Source: CAD feature listing. Evaluate the final solid. Frame: model axes, mm. A direction names the side the tool comes from. Give positions to 0.01 mm unless a question says otherwise; leave off trailing zeros. Write item = value, one per line.
from build123d import *

# Parameters (mm, degrees)
BOSS_EXTRUDE1_DEPTH = 63
CUT_EXTRUDE4_DEPTH  = 60
BOSS_EXTRUDE5_DEPTH = 5
FILLET3_R           = 5
BOSS_EXTRUDE6_DEPTH = 5
BOSS_EXTRUDE7_DEPTH = 63
FILLET4_R           = 5
SKETCH14_R          = 1.9999999999999996
SKETCH14_R_2        = 2
CUT_EXTRUDE5_DEPTH  = 10
SKETCH15_R          = 4.000000000000002
SKETCH15_R_2        = 2
SKETCH15_R_3        = 4.000000000000001
SKETCH15_R_4        = 1.9999999999999996
BOSS_EXTRUDE8_DEPTH = 5
CUT_EXTRUDE6_START  = -5
SKETCH16_R          = 2
SKETCH16_R_2        = 1.9999999999999996
CUT_EXTRUDE6_DEPTH  = 5


# Read off the part's stored shape, not the designer's step: Boss-Extrude1
with BuildPart() as part:
    # Boss-Extrude1 outline → Boss-Extrude1 (new body)
    with BuildSketch(Plane.XY):
        with BuildLine():
            Line((4.954113003, -60.810475982), (9.954113003, -60.810475982))
            add(Edge.make_bspline(
                [(9.954113003, -60.810475982), (1.78782004145555, -34.5665002552168), (-27.9913048539535, -7.28206006884536), (-18.045886997, 21.189524018)],
                knots=[0, 0, 0, 0, 1, 1, 1, 1], degree=3))
            Line((-18.045886997, 21.189524018), (-23.045886997, 21.189524018))
            add(Edge.make_bspline(
                [(-23.045886997, 21.189524018), (-23.192896954450642, 20.707388183877445), (-23.619107908159766, 19.212032019757164), (-24.3984566732412, 15.7227335791878), (-24.9259424602794, 10.7154717202631), (-24.7059244457818, 4.80639957244901), (-23.4437954980132, -2.90791828688786), (-20.3649701079, -12.2138739410152), (-15.1627192062184, -22.9267758821705), (-9.22446854976525, -33.2839412268649), (-4.2731817504284, -41.6523064711653), (-0.670405229165687, -48.1782991582584), (1.76514247549924, -52.980809675903), (3.49961876568494, -56.8892897902748), (4.492016037450547, -59.4867262662843), (4.856824135774904, -60.5259563871115), (4.954113003, -60.810475982)],
                knots=[0.01630237867055594, 0.01630237867055594, 0.01630237867055594, 0.01630237867055594, 0.03125, 0.0625, 0.125, 0.1875, 0.25, 0.375, 0.5, 0.625, 0.75, 0.8125, 0.875, 0.9375, 0.96875, 0.9805431413660037, 0.9805431413660037, 0.9805431413660037, 0.9805431413660037], degree=3))
        make_face()
    extrude(amount=BOSS_EXTRUDE1_DEPTH)

    # Sketch10 → Cut-Extrude4 (cut)
    with BuildSketch(Plane.XZ.offset(60.81047598214444)):
        with BuildLine():
            Line((9.954113003304059, 63), (9.954113003304059, 44.66190378968828))
            ThreePointArc((9.954113003304059, 44.66190378968828), (4.065539070195477, 55.13527900478137), (-5.018130619372688, 63))
            Line((-5.018130619372688, 63), (4.954113003304057, 63))
            Line((4.954113003304057, 63), (9.954113003304059, 63))
        make_face()
    extrude(amount=-CUT_EXTRUDE4_DEPTH, mode=Mode.SUBTRACT)

    # Sketch11 → Boss-Extrude5 (add)
    with BuildSketch(Plane.XZ.offset(60.81047598214444)):
        with BuildLine():
            Line((-15.045886996695936, 6e-16), (4.954113003304057, 0))
            Line((4.954113003304057, 0), (4.954113003304058, 54.00000000000057))
            ThreePointArc((4.954113003304058, 54.00000000000057), (0.4038163976446967, 58.98290612532635), (-5.018130619372695, 63))
            Line((-5.018130619372695, 63), (-15.045886996695936, 63))
            Line((-15.045886996695936, 63), (-15.045886996695936, 6e-16))
        make_face()
    extrude(amount=-BOSS_EXTRUDE5_DEPTH)

    # Fillet3
    fillet3_edges = [part.edges().sort_by_distance(p)[0] for p in [
        (3.003762593217399, -55.81047598214444, 28.187768789799662),
    ]]
    fillet(fillet3_edges, radius=FILLET3_R)



with BuildPart() as body_2:
    # Sketch12 → Boss-Extrude6 (new body)
    with BuildSketch(Plane(origin=(0, 21.189524017855575, 0), x_dir=(1, 0, 0), z_dir=(0, 1, 0))):
        Polygon((-18.04588699669594, -63), (-18.04588699669594, 0), (-8.045886996695941, -3.31e-15), (-8.045886996695941, -63), align=None)
    extrude(amount=-BOSS_EXTRUDE6_DEPTH)


with BuildPart() as part_1:
    add(part.part)

    add(body_2.part)  # Boss-Extrude7 merges body 2
    # Sketch13 → Boss-Extrude7 (add)
    with BuildSketch(Plane.XY.offset(63)):
        with BuildLine():
            Line((-18.04588699669594, 16.189524017855575), (-18.04588699669594, 21.189524017855575))
            add(Edge.make_bspline(
                [(-19.398734896011995, 16.18952401785558), (-19.076313221090718, 17.852122543862073), (-18.62949534090365, 19.51877933077492), (-18.04588699669594, 21.189524017855575)],
                knots=[0.9413188714055053, 0.9413188714055053, 0.9413188714055053, 0.9413188714055053, 1, 1, 1, 1], degree=3))
            Line((-19.398734896011995, 16.18952401785558), (-18.04588699669594, 16.189524017855575))
        make_face()
    extrude(amount=-BOSS_EXTRUDE7_DEPTH)

    # Fillet4
    fillet4_edges = [part_1.edges().sort_by_distance(p)[0] for p in [
        (-19.398734896011995, 16.18952401785558, 31.5),
    ]]
    fillet(fillet4_edges, radius=FILLET4_R)

    # Sketch14 → Cut-Extrude5 (cut)
    with BuildSketch(Plane.XZ.offset(-16.18952401785553)):
        with Locations((-11.045886996695984, 8)):
            Circle(SKETCH14_R)
        with Locations((-11.045886996695984, 55)):
            Circle(SKETCH14_R_2)
    extrude(amount=-CUT_EXTRUDE5_DEPTH, mode=Mode.SUBTRACT)

    # Sketch15 → Boss-Extrude8 (add)
    # profile 1 of 2: a face of its own
    with BuildSketch(Plane.XZ.offset(-16.18952401785553)):
        with Locations((-11.045886996695982, 55)):
            Circle(SKETCH15_R)
        with Locations((-11.045886996695982, 55)):
            Circle(SKETCH15_R_2, mode=Mode.SUBTRACT)
    # profile 2 of 2: a face of its own
    with BuildSketch(Plane.XZ.offset(-16.18952401785553)):
        with Locations((-11.045886996695982, 8)):
            Circle(SKETCH15_R_3)
        with Locations((-11.045886996695982, 8)):
            Circle(SKETCH15_R_4, mode=Mode.SUBTRACT)
    extrude(amount=-BOSS_EXTRUDE8_DEPTH)

    # Sketch16 → Cut-Extrude6 (cut)
    with BuildSketch(Plane(origin=(0, -55.81047598214444, 0), x_dir=(1, 0, 0), z_dir=(0, 1, 0)).offset(CUT_EXTRUDE6_START)):
        with Locations((-11.045886996695936, -55)):
            Circle(SKETCH16_R)
        with Locations((-11.045886996695936, -8)):
            Circle(SKETCH16_R_2)
    extrude(amount=CUT_EXTRUDE6_DEPTH, mode=Mode.SUBTRACT)


solid = part_1.part
(1) Material intervals for line 1 (Y direction, x = -12.5, z = 44.5); line 2 (Y direction, x = -10.5, z = 59); line 3 (Y direction, x = -8, z = 31.5), sorted ascending.
Values follow:
line_1 = -60.81 to -55.81, -27.52 to -17.41, 16.19 to 21.19
line_2 = -60.81 to -55.81, -31.03 to -21.28, 16.19 to 21.19
line_3 = -60.81 to -55.81, -35.33 to -25.82
(2) Access query for faces 1 (the face through (-7.046, 18.655, 54.96)), 2 (the face through (-9.971, 18.655, 56.686)), 3 (the face through (-8.046, 19, 60)), 4 (the face through (-11, -58, 53)). Directions: +Z, -Z, +X, -X, +Y, -Y. A direction counts if a zero-diameter tool reaches every point of the face in a straight line with its end or side. Return the directions, or none.
Values follow:
face_1 = +X, +Y
face_2 = +Y
face_3 = +Z, +X, +Y
face_4 = -Y
(3) Pull-direction query (X, two-part tool) for faces 5 (the face through (-8.046, 19, 3)), 6 (the face through (-15.046, -58, 32)), 7 (the face through (-13.044, -58.345, 7.912)); classes: pulls with the +X half, pulls with the -X half, needs draft (parallel to the pull), parting line crosses it, or undercut.
Values follow:
face_5 = pulls with the +X half
face_6 = pulls with the -X half
face_7 = undercut
(4) First-contact query: pin 1 (4 mm diameter, centred on y = 19, z = 3.5, fed in from +X); pin 2 (5.5 mm diameter, centred on y = -58.5, z = 45, fed in from -X); pin 3 (10 mm diameter, centred on y = 1.5, z = 54.5, fed in from -X). Flat tips, straight axial feed; report the tip coordinate or a pass-through.
Values follow:
pin_1 = -7.92
pin_2 = -15.05
pin_3 = -24.72
(5) Section query A-A (z = 8). Give the number of separate pieces and of enclosed holes in the cut face, plus the area to 3 significant figures.
Values follow:
separate_pieces = 3
enclosed_holes = 0
area = 556 mm2
